The listing builds one solid part. Answer for the finished solid, in the listing's coordinates (mm). A direction names the side the tool comes from. Round coordinates to 2 decimals unless told otherwise and drop trailing zeros. Write each loop counter-clockwise with the first axis right and the second up, starting at its lowest first coordinate (ties: lowest second). Pieces come first, ordered by that corner, then holes.
(1) The mould has two halves that part along Z. Classify faces 1 (the face through (0, 0, 314.325)), 2 (the face through (-0.9, -5.2, 7.366)), 3 (the face through (-1.38, 6.2, 311.11)): +Z half, -Z half, draft (parallel to the pull), parting line (faces both ways), or undercut.
(2) Each of these flat-tipped pins is pushed along its axis until it touches: pin 1 Ø1.1 at (y, z) = (5.5, 18) entering from +X; pin 2 Ø1.5 at (y, z) = (5.5, 296.5) entering from -X; pin 3 Ø1 at (y, z) = (-2.5, 139.5) entering from +X. Where does it stop, or does it pass through?
(3) A cutting plane is placed at A-A, the plane y = 2. Give the vertices of the cut face in (x, z) (3 decimals), and give its area (3 significant figures).
(4) A cutting plane is placed at B-B, the plane z = 157.5. Give the vertices of the cut face in (x, y), and give its area (3 significant figures).
(5) For faces 4 (the face through (-2, 5, 6.35)), 5 (the face through (-0.8, -6.3, 155.1)), determine the directions among +Z, -Z, +X, -X, +Y, -Y from which every point of the face is accessible in a straight line to the end or side of a thin tool.
(6) Find the intervals of material crossed by probe 1 along Z at (x, y) = (2.5, -4.5) (3 decimals); probe 2 along X at (y, z) = (-0.75, 73); probe 3 along X at (y, z) = (2.25, 56), in increasing order.
Autodesk Inventor part; units mm, degrees
ref_plane "Work Plane1" through (0, 6.35, 0) normal (0, 1, 0) x (-1, 0, 0)
ref_plane "Work Plane2" through (6.35, 6.35, 307.975) normal (0, 0, 1) x (1, 0, 0)
ref_plane "Work Plane3" through (6.35, 6.35, 6.35) normal (0, 0, -1) x (-1, 0, 0)
sketch "Sketch1" plane through (0, 0, 0) normal (0, 0, 1) x (1, 0, 0)
  circle A0 centre (0, 0) radius 6.35
  dimension "d0" = 12.7
extrude "Extrusion1" add sketch "Sketch1" along normal blind 314.325
ref_plane "Work Plane1" through (0, 6.35, 0) normal (0, 1, 0) x (-1, 0, 0)
sketch "Sketch2" plane through (0, 6.35, 0) normal (0, 1, 0) x (-1, 0, 0)
  line L0 (-6.35, 314.325) -> (6.35, 314.325)
  line L1 (-6.35, 0) -> (6.35, 0)
  line L2 (-6.35, 0) -> (-6.35, 314.325)
  line L3 (6.35, 0) -> (6.35, 314.325)
  line L4 (-6.35, 6.35) -> (6.35, 6.35)
  line L5 (-6.35, 307.975) -> (6.35, 307.975)
  arc A0 (1.5875, 306.3875) -> (-1.5875, 306.3875) centre (0, 306.3875) ccw
  line L6 (-1.5875, 306.3875) -> (-1.5875, 287.3375)
  line L7 (1.5875, 306.3875) -> (1.5875, 287.3375)
  arc A1 (-1.5875, 287.3375) -> (1.5875, 287.3375) centre (0, 287.3375) ccw
  arc A2 (1.5875, 26.9875) -> (-1.5875, 26.9875) centre (0, 26.9875) ccw
  line L8 (-1.5875, 26.9875) -> (-1.5875, 7.9375)
  line L9 (1.5875, 26.9875) -> (1.5875, 7.9375)
  arc A3 (-1.5875, 7.9375) -> (1.5875, 7.9375) centre (0, 7.9375) ccw
  point P0 (0, 0)
  dimension "d3" = 301.625
  dimension "d4" = 6.35
  dimension "d5" = 6.35
  dimension "d11" = 19.05
  dimension "d12" = 3.175
  dimension "d13" = 19.05
  dimension "d14" = 3.175
  dimension "d15" = 7.9375
  dimension "d16" = 279.4
  dimension "d17" = 6.35
ref_plane "Work Plane2" through (6.35, 6.35, 307.975) normal (0, 0, 1) x (1, 0, 0)
ref_plane "Work Plane3" through (6.35, 6.35, 6.35) normal (0, 0, -1) x (-1, 0, 0)
sketch "Sketch3" plane through (6.35, 6.35, 307.975) normal (0, 0, 1) x (1, 0, 0)
  circle A0 centre (-6.35, -6.35) radius 6.35
  circle A1 centre (-6.35, -6.35) radius 5.08
  dimension "d6" = 10.16
extrude "Extrusion2" cut sketch "Sketch3" against normal blind 1.016
sketch "Sketch4" plane through (6.35, 6.35, 6.35) normal (0, 0, -1) x (-1, 0, 0)
  circle A0 centre (6.35, -6.35) radius 5.08
  circle A1 centre (6.35, -6.35) radius 6.35
extrude "Extrusion3" cut sketch "Sketch4" against normal blind 1.016
extrude "Extrusion4" cut sketch "Sketch2" against normal blind 1.5875 contours A3 L8 A2 L9 | A0 L7 A1 L6
equation "\"d4\" = d5"
properties part number "8 ball roller shaft"
Solutions:
1. face 1: +Z half
1. face 2: undercut
1. face 3: draft
2. pin 1: stops at x = 3.98
2. pin 2: stops at x = -4.21
2. pin 3: stops at x = 6.03
3. outline: (-6.027, 0) - (6.027, 0) - (6.027, 6.35) - (4.67, 6.35) - (4.67, 7.366) - (6.027, 7.366) - (6.027, 306.959) - (4.67, 306.959) - (4.67, 307.975) - (6.027, 307.975) - (6.027, 314.325) - (-6.027, 314.325) - (-6.027, 307.975) - (-4.67, 307.975) - (-4.67, 306.959) - (-6.027, 306.959) - (-6.027, 7.366) - (-4.67, 7.366) - (-4.67, 6.35) - (-6.027, 6.35) - close
3. area: 3,780 mm2
4. outline: circle Ø12.7 at (0, 0)
4. area: 127 mm2
5. face 4: none
5. face 5: +Z, -Z
6. probe 1: z = 0 to 6.35, 7.366 to 306.959, 307.975 to 314.325
6. probe 2: x = -6.31 to 6.31
6. probe 3: x = -5.94 to 5.94
